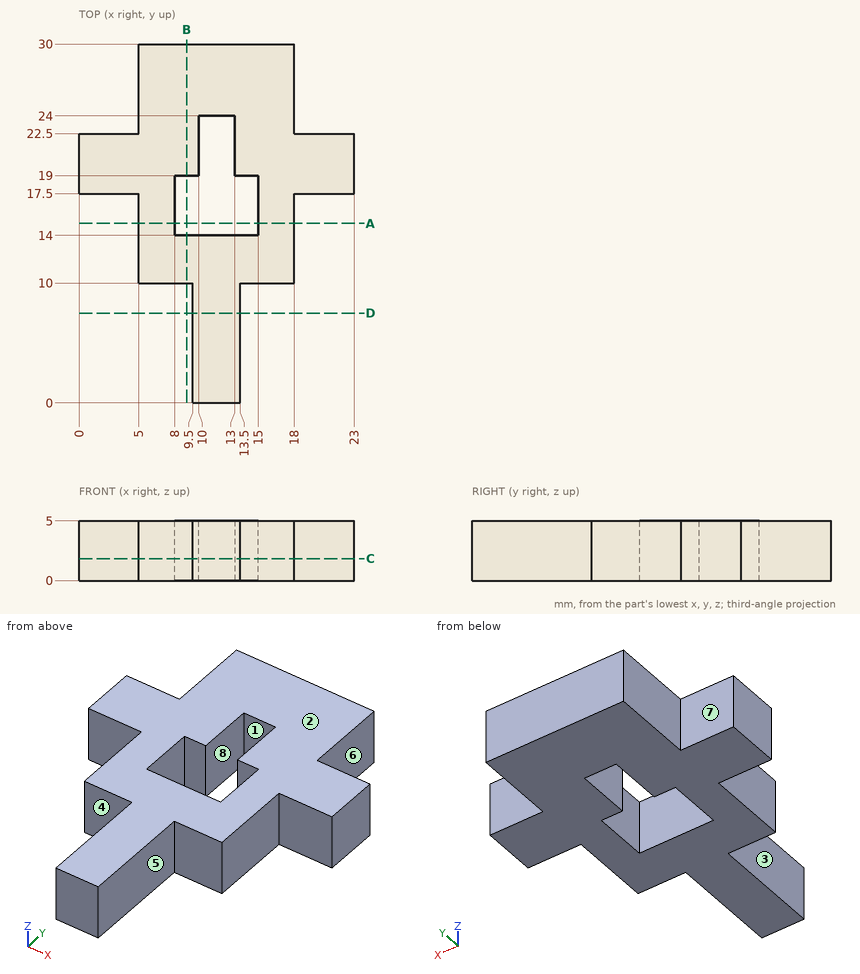
Study the drawing (mm; zero at the part's minimum x, y, z) and answer. A direction names the side the tool comes from. Coordinates: 2 decimals unless noted, no trailing zeros. Write each loop counter-clockwise with the first axis right and the second up, starting at its lowest first coordinate (ties: lowest second). Pieces come first, ordered by that corner, then holes. Notation, with made-up numbers: (-5, 15) - (34, 15) arc R35 cw to (34, 53) - close; hole circle Ø9 at (14, 58). An arc over 180 degrees is marked (long way). Return JSON: item names as keys, results as strings. Group by question number.
1. Which of the six approach directions +Z, -Z, +X, -X, +Y, -Y give full straight-line access (tool end or side, diameter ignored) to the marked faces 4, 5, 6, 7 and 8?
2. A cutting plane is placed at C-C, the plane z = 1.85. Determine the outline of the cut face in (x, y), plus the area to 3 significant figures.
3. Straight lines are drawn through the part: L1, parallel to X at y = 18.75, z = 2.4; L2, parallel to X at y = 20.25, z = 3.6; L3, parallel to Y at x = 18.25, z = 2.4. For each, find the intervals that lie inside material, in ascending order.
4. Determine the mould class of the marked faces 1, 2 and 3 for opening direction X: released by +X, released by -X, zero draft, split by the parting line, or undercut.
5. Given pin 1 (1 mm diameter, centred on y = 24, z = 4.5, fed in from -X); pin 2 (2.5 mm diameter, centred on y = 3, z = 3, fed in from -X); pin 3 (3 mm diameter, centred on y = 25.5, z = 3, fed in from +X), each flat-ended and moving along its own axis, determine where each tip first touches the part or whether it passes through.
6. A cutting plane is placed at A-A, the plane y = 15. Determine the outline of the cut face in (x, z), plus the area to 3 significant figures.
7. A cutting plane is placed at D-D, the plane y = 7.5. Determine the outline of the cut face in (x, z), plus the area to 3 significant figures.
8. A cutting plane is placed at B-B, the plane x = 9. Determine the outline of the cut face in (y, z).
Ans:
{
 "1": {"face 4": "+Z, -Z, -X, -Y", "face 5": "+Z, -Z, +X, -Y", "face 6": "+Z, -Z, +X, +Y", "face 7": "+Z, -Z, -X, +Y", "face 8": "+Z, -Z"},
 "2": {"outline": "(0, 17.5) - (5, 17.5) - (5, 10) - (9.5, 10) - (9.5, 0) - (13.5, 0) - (13.5, 10) - (18, 10) - (18, 17.5) - (23, 17.5) - (23, 22.5) - (18, 22.5) - (18, 30) - (5, 30) - (5, 22.5) - (0, 22.5) - close; hole (8, 14) - (15, 14) - (15, 19) - (13, 19) - (13, 24) - (10, 24) - (10, 19) - (8, 19) - close", "area": "300 mm²"},
 "3": {"L1": "0 to 8, 15 to 23", "L2": "0 to 10, 13 to 23", "L3": "17.5 to 22.5"},
 "4": {"face 1": "undercut", "face 2": "zero draft", "face 3": "released by -X"},
 "5": {"pin 1": "x = 5", "pin 2": "x = 9.5", "pin 3": "x = 18"},
 "6": {"outline": "(5, 0) - (8, 0) - (8, 5) - (5, 5) - close; (15, 0) - (18, 0) - (18, 5) - (15, 5) - close", "area": "30.0 mm²"},
 "7": {"outline": "(9.5, 0) - (13.5, 0) - (13.5, 5) - (9.5, 5) - close", "area": "20.0 mm²"},
 "8": {"outline": "(10, 0) - (14, 0) - (14, 5) - (10, 5) - close; (19, 0) - (30, 0) - (30, 5) - (19, 5) - close"}
}
